Source: CAD feature listing. Evaluate the final solid. Frame: model axes, mm. Coordinates: 2 decimals unless noted, no trailing zeros. Loops run counter-clockwise (first coordinate to the right, second up) from the corner with the lowest first, then second, coordinate; pieces in that order, holes last. Notation, with made-up numbers: (-38.5, 20) -> (-20.5, 20) arc R24 cw to (-20.5, 55) -> close; hole circle Ø8 at (79, 11.25). An arc over 180 degrees is marked (long way). Answer as CSV lines item,"result".
from build123d import *

# Parameters (mm, degrees)
SKETCH1_R           = 22.5
SKETCH1_R_2         = 4
SKETCH1_R_3         = 1.5
BOSS_EXTRUDE1_DEPTH = 5


with BuildPart() as part:
    # Sketch1 → Boss-Extrude1 (new body)
    with BuildSketch(Plane(origin=(0, 0, 0), x_dir=(0, 0, -1), z_dir=(1, 0, 0))):
        Circle(SKETCH1_R)
        Circle(SKETCH1_R_2, mode=Mode.SUBTRACT)
        with Locations((-10.606601718, 10.606601718)):
            Circle(SKETCH1_R_3, mode=Mode.SUBTRACT)
        with Locations(Location((-10.606601718, -10.606601718, 0), (0, 0, 180))):
            Circle(SKETCH1_R_3, mode=Mode.SUBTRACT)
        with Locations((10.606601718, -10.606601718)):
            Circle(SKETCH1_R_3, mode=Mode.SUBTRACT)
        with Locations((10.606601718, 10.606601718)):
            Circle(SKETCH1_R_3, mode=Mode.SUBTRACT)
    extrude(amount=BOSS_EXTRUDE1_DEPTH)


solid = part.part
(1) Material intervals for L1, parallel to Z at x = 4.6, y = -10.5; L2, parallel to Z at x = 0.9, y = -11; L3, parallel to Y at x = 0.75, z = 10, sorted ascending. Write a range as [from, to].
Computed values:
L1,"[-19.9, -12.1], [-9.11, 9.11], [12.1, 19.9]"
L2,"[-19.63, -12.05], [-9.16, 9.16], [12.05, 19.63]"
L3,"[-20.16, -11.98], [-9.23, 9.23], [11.98, 20.16]"
(2) Cut plane A-A (y = 0). Return the cut outline in (x, z), then the cut area to 3 significant figures.
Computed values:
outline,"(0, -22.5) -> (5, -22.5) -> (5, -4) -> (0, -4) -> close; (0, 4) -> (5, 4) -> (5, 22.5) -> (0, 22.5) -> close"
area,"185 mm^2"
(3) Cut plane D-D (x = 4.35). Return the cut outline in (y, z), then the cut area to 3 significant figures.
Computed values:
outline,"circle Ø45 at (0, 0); hole circle Ø3 at (-10.61, -10.61); hole circle Ø3 at (-10.61, 10.61); hole circle Ø8 at (0, 0); hole circle Ø3 at (10.61, -10.61); hole circle Ø3 at (10.61, 10.61)"
area,"1,510 mm^2"
(4) Pin query (flat end, axial travel): pin 1 Ø1.5 at (x, z) = (4.5, 5) entering from +Y; pin 2 Ø1.5 at (x, z) = (2.5, -0.5) entering from +Y; pin 3 Ø2 at (x, y) = (3, 1.5) entering from -Z; pin 4 Ø5 at (y, z) = (0, 0) entering from +X. Return the tip coordinate at first contact, or that it passes through.
Computed values:
pin 1,"y = 22.09"
pin 2,"y = 22.5"
pin 3,"z = -22.49"
pin 4,"through"
(5) Cut plane C-C (y = -11.5). Return the cut outline in (x, z), then the cut area to 3 significant figures.
Computed values:
outline,"(0, -19.34) -> (5, -19.34) -> (5, -11.81) -> (0, -11.81) -> close; (0, -9.4) -> (5, -9.4) -> (5, 9.4) -> (0, 9.4) -> close; (0, 11.81) -> (5, 11.81) -> (5, 19.34) -> (0, 19.34) -> close"
area,"169 mm^2"
(6) Draft query along Y for faces 1 (the flat face through (5, -5, 0)), 2 (the cylindrical face through (2.465, -19.961, -10.382)), 3 (the cylindrical face through (2.465, -3.905, 0.867)). Return one class per face: released by +Y, released by -Y, zero draft, split by the parting line, or undercut.
Computed values:
face 1,"zero draft"
face 2,"split by the parting line"
face 3,"undercut"
